Check sheet for the modelled part. Datum: model origin and axes. Units: mm. Face numbers are marked on the shaded views. A direction names the side the tool comes from. Round coordinates to 2 decimals unless told otherwise and drop trailing zeros. Write each loop counter-clockwise with the first axis right and the second up, starting at its lowest first coordinate (ties: lowest second). Pieces come first, ordered by that corner, then holes. Notation, with made-up numbers: (89, 78.5) -> (113, 78.5) arc R26 cw to (113, 115.5) -> close; hole circle Ø4 at (-6, -25). An arc over 180 degrees is marked (long way). One line per item, written item: value.
from build123d import *

# Parameters (mm, degrees)
SM_BASE_FLANGE_1_DEPTH = 30
CUT_EXTRUDE_1_REACH    = 43.476
SKETCH_6_R             = 5.55
CUT_EXTRUDE_2_REACH    = 49.896
SKETCH_7_R             = 2.1
CHAMFER_1_SIZE         = 5


# Sheet-metal steps are written as plain solids
with BuildPart() as part:
    # Sketch 1 → 基材-凸緣1 (new body)
    with BuildSketch(Plane.XY):
        with BuildLine():
            Line((-10, 17.5), (-10, -16.7634))
            ThreePointArc((-10, -16.7634), (-9.784254855, -17.284254855), (-9.2634, -17.5))
            Line((-9.2634, -17.5), (10, -17.5))
            Line((10, -17.5), (10, -20.5))
            Line((10, -20.5), (-9.2634, -20.5))
            ThreePointArc((-9.2634, -20.5), (-11.905575199, -19.405575199), (-13, -16.7634))
            Line((-13, -16.7634), (-13, 17.5))
            Line((-13, 17.5), (-10, 17.5))
        make_face()
    extrude(amount=SM_BASE_FLANGE_1_DEPTH)

    # 草圖6 → 除料-伸長1 (cut, up to next)
    with BuildSketch(Plane(origin=(-10, 0, 0), x_dir=(0, 0, -1), z_dir=(1, 0, 0)), mode=Mode.PRIVATE) as cut_extrude_1_sk1:
        with Locations(Location((-15, 0.75, 0), (0, 0, 90))):
            Circle(SKETCH_6_R)
    cut_extrude_1_tool1 = extrude(cut_extrude_1_sk1.sketch, amount=-CUT_EXTRUDE_1_REACH, mode=Mode.PRIVATE) & part.part
    add(cut_extrude_1_tool1.solids().sort_by_distance((-10, 0.75, 15))[0], mode=Mode.SUBTRACT)

    # 草圖7 → 除料-伸長2 (cut, up to next)
    with BuildSketch(Plane(origin=(0, -17.5, 0), x_dir=(1, 0, 0), z_dir=(0, 1, 0)), mode=Mode.PRIVATE) as cut_extrude_2_sk1:
        with Locations(Location((0.3683, -22.5, 0), (0, 0, 270))):
            Circle(SKETCH_7_R)
    cut_extrude_2_tool1 = extrude(cut_extrude_2_sk1.sketch, amount=-CUT_EXTRUDE_2_REACH, mode=Mode.PRIVATE) & part.part
    # 草圖7 → 除料-伸長2 (cut, up to next)
    with BuildSketch(Plane(origin=(0, -17.5, 0), x_dir=(1, 0, 0), z_dir=(0, 1, 0)), mode=Mode.PRIVATE) as cut_extrude_2_sk2:
        with Locations(Location((0.3683, -7.5, 0), (0, 0, 270))):
            Circle(SKETCH_7_R)
    cut_extrude_2_tool2 = extrude(cut_extrude_2_sk2.sketch, amount=-CUT_EXTRUDE_2_REACH, mode=Mode.PRIVATE) & part.part
    add(cut_extrude_2_tool1.solids().sort_by_distance((0.3683, -17.5, 22.5))[0], mode=Mode.SUBTRACT)
    add(cut_extrude_2_tool2.solids().sort_by_distance((0.3683, -17.5, 7.5))[0], mode=Mode.SUBTRACT)

    # 導角1
    chamfer_1_edges = [part.edges().sort_by_distance(p)[0] for p in [
        (-11.5, 17.5, 30),
        (-11.5, 17.5, 0),
        (10, -19, 30),
        (10, -19, 0),
    ]]
    chamfer(chamfer_1_edges, length=CHAMFER_1_SIZE)


solid = part.part
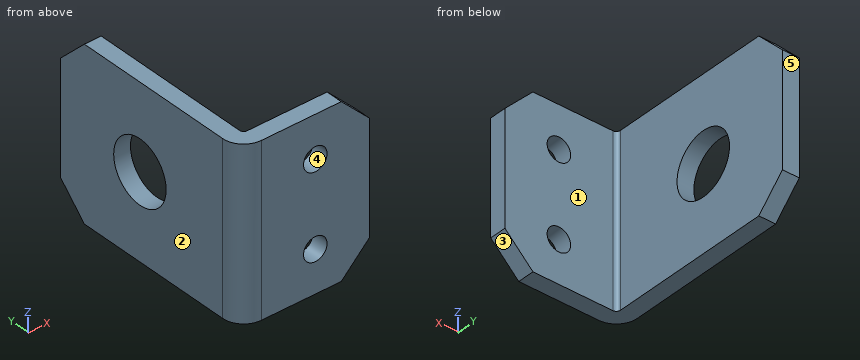
Item 1: Sectioned sample at B-B on y = 0.75. Enter the section's corners in (x, z).
Answer:
outline: (-13, 0) -> (-10, 0) -> (-10, 9.45) -> (-13, 9.45) -> close; (-13, 20.55) -> (-10, 20.55) -> (-10, 30) -> (-13, 30) -> close
Item 2: Thickness scan on line 1 (Z direction, x = -11.6, y = 0.75); line 2 (Y direction, x = -9.25, z = 2.25); line 3 (X direction, y = -19.75, z = 7.5). Record the ranges inside material, lowest first.
Answer:
line 1: z = 0 to 9.45, 20.55 to 30
line 2: y = -20.5 to -17.5
line 3: x = -11.51 to -1.73, 2.47 to 10
Item 3: Sectioned sample at C-C on z = 22.5. Enter the section's corners in (x, y).
Answer:
outline: (-13, -16.76) arc R3.74 ccw to (-9.26, -20.5) -> (-1.73, -20.5) -> (-1.73, -17.5) -> (-9.26, -17.5) arc R0.74 cw to (-10, -16.76) -> (-10, 17.5) -> (-13, 17.5) -> close; (2.47, -20.5) -> (10, -20.5) -> (10, -17.5) -> (2.47, -17.5) -> close
Item 4: Sectioned sample at D-D on y = 14. Enter the section's corners in (x, z), and give its area (3 significant figures).
Answer:
outline: (-13, 1.5) -> (-10, 1.5) -> (-10, 28.5) -> (-13, 28.5) -> close
area: 81.0 mm^2
Item 5: Depth check by flat-ended pin: P1, Ø2, axis at y = -9.5, z = 24, coming from the +X side; P2, Ø5.5, axis at x = 0.37, z = 7.5, coming from the +Y side. Enter the tip coordinate at first touch or a pass-through.
Answer:
P1: stops at x = -10
P2: stops at y = -17.5
Item 6: Mould release check, pull along Z, two halves, no side actions. Record for the marked faces 3, 4 and 5: pulls with the +Z half, pulls with the -Z half, needs draft (parallel to the pull), parting line crosses it, or undercut.
Answer:
face 3: pulls with the -Z half
face 4: undercut
face 5: needs draft
Item 7: Sectioned sample at A-A on z = 15. Enter the section's corners in (x, y).
Answer:
outline: (-13, -16.76) arc R3.74 ccw to (-9.26, -20.5) -> (10, -20.5) -> (10, -17.5) -> (-9.26, -17.5) arc R0.74 cw to (-10, -16.76) -> (-10, -4.8) -> (-13, -4.8) -> close; (-13, 6.3) -> (-10, 6.3) -> (-10, 17.5) -> (-13, 17.5) -> close
Item 8: Tool access check on the marked faces 1 and 2. Record the directions out of +Z, -Z, +X, -X, +Y, -Y that give a thin tool (end or side, any length) a straight path to the whole face; none if there is none.
Answer:
face 1: +Z, -Z, +X, +Y
face 2: +Z, -Z, -X, +Y, -Y
